from build123d import *

# Parameters (mm, degrees)
EXTRUDE_THIN1_DEPTH            = 6
CBORE_FOR_M4_SHCS1_D           = 4.5
CBORE_FOR_M4_SHCS1_CBORE_D     = 8
CBORE_FOR_M4_SHCS1_CBORE_DEPTH = 4


with BuildPart() as part:
    # Sketch1 → Extrude-Thin1 (new body)
    with BuildSketch(Plane(origin=(0, 0, 0), x_dir=(1, 0, 0), z_dir=(0, 1, 0))):
        Polygon((-162.4, 80), (0, 80), (0, -80), (-162.4, -80), (-162.4, -40), (-40, -40), (-40, 40), (-162.4, 40), align=None)
    extrude(amount=EXTRUDE_THIN1_DEPTH)

    # CBORE for M4 SHCS1 (through all)
    with Locations(Plane(origin=(0, 6, 0), x_dir=(1, 0, 0), z_dir=(0, 1, 0))):
        with Locations((-20, -60), (-142.4, 60), (-142.4, -60), (-20, 60)):
            CounterBoreHole(CBORE_FOR_M4_SHCS1_D / 2, CBORE_FOR_M4_SHCS1_CBORE_D / 2, CBORE_FOR_M4_SHCS1_CBORE_DEPTH)


solid = part.part
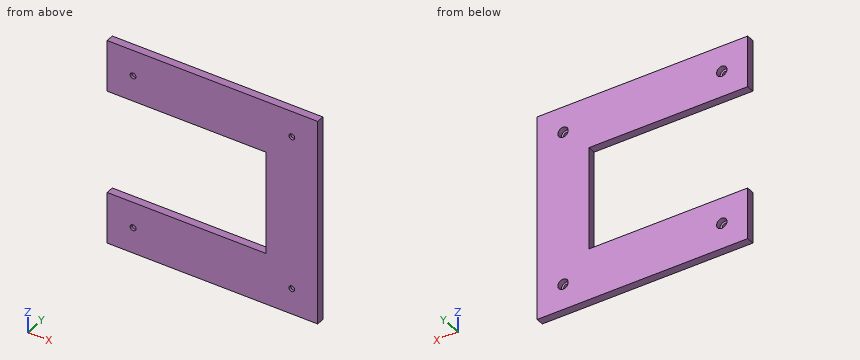
Source: CAD feature listing. Evaluate the final solid. Frame: model axes, mm. Give positions to 0.01 mm unless a question says otherwise; leave off trailing zeros. Write each loop counter-clockwise with the first axis right and the second up, starting at its lowest first coordinate (ties: lowest second). Pieces come first, ordered by that corner, then holes. Notation, with made-up numbers: (-10.5, 5) -> (29.5, 5) arc R22 ccw to (29.5, 16) -> close; hole circle Ø9 at (13, 55.25). An arc over 180 degrees is marked (long way). Write item = value, one per line.
Q1. First-contact query: pin 1 (10.5 mm diameter, centred on x = -20, z = -60, fed in from +Y); pin 2 (3.5 mm diameter, centred on x = -142.4, z = 60, fed in from -Y); pin 3 (7 mm diameter, centred on x = -142.4, z = -60, fed in from +Y). Flat tips, straight axial feed; report the tip coordinate or a pass-through.
Here are the results:
pin_1 = 6
pin_2 = through
pin_3 = 2
Q2. Line query: line 1 (Z direction, x = -142.4, y = 1.25); line 2 (X direction, y = 3.6, z = 60); line 3 (Z direction, x = -20, y = 3.75). Output: solid intervals per line, ascending. Write a range as from..to.
Here are the results:
line_1 = -80..-62.25, -57.75..-40, 40..57.75, 62.25..80
line_2 = -162.4..-146.4, -138.4..-24, -16..0
line_3 = -80..-64, -56..56, 64..80
Q3. Cut plane C-C on x = -142.4. Return loops of the section in (y, z).
Here are the results:
outline = (0, -80) -> (6, -80) -> (6, -64) -> (2, -64) -> (2, -62.25) -> (0, -62.25) -> close; (0, -57.75) -> (2, -57.75) -> (2, -56) -> (6, -56) -> (6, -40) -> (0, -40) -> close; (0, 40) -> (6, 40) -> (6, 56) -> (2, 56) -> (2, 57.75) -> (0, 57.75) -> close; (0, 62.25) -> (2, 62.25) -> (2, 64) -> (6, 64) -> (6, 80) -> (0, 80) -> close
Q4. Cut plane D-D on y = 5.1. Return loops of the section in (x, z), then the cut area to 3 significant figures.
Here are the results:
outline = (-162.4, -80) -> (0, -80) -> (0, 80) -> (-162.4, 80) -> (-162.4, 40) -> (-40, 40) -> (-40, -40) -> (-162.4, -40) -> close; hole circle Ø8 at (-142.4, -60); hole circle Ø8 at (-142.4, 60); hole circle Ø8 at (-20, -60); hole circle Ø8 at (-20, 60)
area = 16,000 mm²
Q5. Cut plane B-B on z = 60. Return loops of the section in (x, y).
Here are the results:
outline = (-162.4, 0) -> (-144.65, 0) -> (-144.65, 2) -> (-146.4, 2) -> (-146.4, 6) -> (-162.4, 6) -> close; (-140.15, 0) -> (-22.25, 0) -> (-22.25, 2) -> (-24, 2) -> (-24, 6) -> (-138.4, 6) -> (-138.4, 2) -> (-140.15, 2) -> close; (-17.75, 0) -> (0, 0) -> (0, 6) -> (-16, 6) -> (-16, 2) -> (-17.75, 2) -> close
Q6. Cut plane A-A on x = -20. Return loops of the section in (y, z).
Here are the results:
outline = (0, -80) -> (6, -80) -> (6, -64) -> (2, -64) -> (2, -62.25) -> (0, -62.25) -> close; (0, -57.75) -> (2, -57.75) -> (2, -56) -> (6, -56) -> (6, 56) -> (2, 56) -> (2, 57.75) -> (0, 57.75) -> close; (0, 62.25) -> (2, 62.25) -> (2, 64) -> (6, 64) -> (6, 80) -> (0, 80) -> close
